Design review of the part shown in the three views and the two pictorial views. Dimensions are in mm from the part's minimum x, y and z. A direction names the side the tool comes from. Give positions to 0.01 mm unless a question says otherwise; leave off trailing zeros. Order: outer loops, then holes, each group sorted by start corner. A loop starts at its lowest first (then second) coordinate and runs counter-clockwise, first axis right, second up. Notation, with made-up numbers: (5.5, 54) - (43.5, 54) arc R35 cw to (43.5, 92) - close; hole circle Ø9 at (54, 58.25). An arc over 180 degrees is marked (long way). Put each result on its own line as item: value.
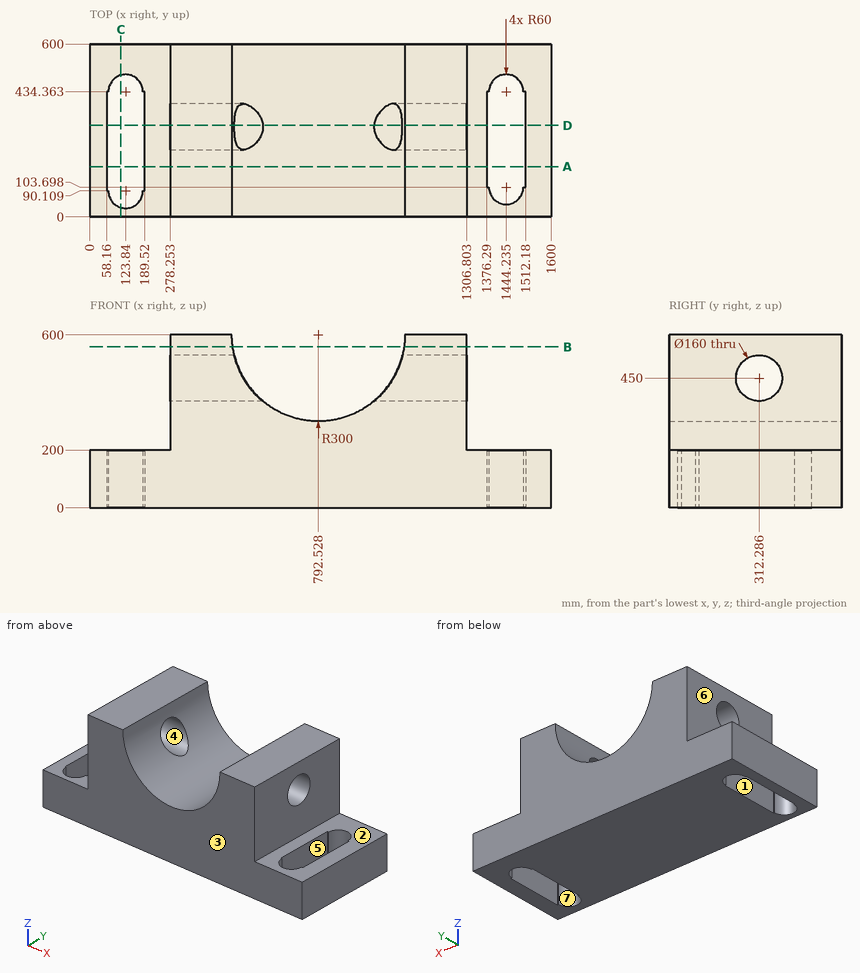
(1) For the marked faces 1, 2 and 3, list the 3-axis set-ups (+Z, -Z, +X, -X, +Y, -Y) from which the entire face can be reached by the end or side of a thin tool; tool diameter is ignored.
The answers:
face 1: +Z, -Z
face 2: +Z, +X, +Y, -Y
face 3: +Z, -Z, +X, -X, -Y
(2) Take a section at D-D, the plane y = 318. Write out the cut boundary in (x, z) (1 decimal), then the cut area to 3 significant figures.
The answers:
outline: (0, 0) - (58.2, 0) - (58.2, 200) - (0, 200) - close; (189.5, 0) - (1376.3, 0) - (1376.3, 200) - (1306.8, 200) - (1306.8, 370.2) - (985.4, 370.2) arc R300 cw to (599.7, 370.2) - (278.3, 370.2) - (278.3, 200) - (189.5, 200) - close; (278.3, 529.8) - (500.9, 529.8) arc R300 cw to (492.5, 600) - (278.3, 600) - close; (1084.2, 529.8) - (1306.8, 529.8) - (1306.8, 600) - (1092.5, 600) arc R300 cw to start; (1512.2, 0) - (1600, 0) - (1600, 200) - (1512.2, 200) - close
area: 454,000 mm^2
(3) Take a section at C-C, the plane x = 107. Write out the cut boundary in (y, z).
The answers:
outline: (0, 0) - (32.52, 0) - (32.52, 200) - (0, 200) - close; (491.95, 0) - (600, 0) - (600, 200) - (491.95, 200) - close
(4) Wall thickness on L1, parallel to X at y = 384, z = 186.5; L2, parallel to Y at x = 358, z = 450; L3, parallel to Y at x = 1440.5, z = 89.5 (1 decimal): over which ranges is each line inside the solid? List them lowest first.
The answers:
L1: 0 to 58.16, 189.52 to 1376.29, 1512.18 to 1600
L2: 0 to 232.29, 392.29 to 600
L3: 0 to 43.8, 494.2 to 600
(5) Take a section at B-B, the plane z = 558.5. Write out the cut boundary in (x, y), then the cut area to 3 significant figures.
The answers:
outline: (278.25, 0) - (495.41, 0) - (495.41, 600) - (278.25, 600) - close; (1089.64, 0) - (1306.8, 0) - (1306.8, 600) - (1089.64, 600) - close
area: 261,000 mm^2
(6) Clearance check with flat-ended pins moving along their axes: pin 1 Ø6 at (y, z) = (356, 281.5) entering from +X; pin 2 Ø3 at (y, z) = (169, 219.5) entering from -X; pin 3 Ø6 at (x, y) = (695.5, 157.5) entering from +Z. State where each tip first meets the part, or that it passes through.
The answers:
pin 1: x = 1306.8
pin 2: x = 278.25
pin 3: z = 317.17
(7) The part is to be moulded in two halves that separate along X. For the marked faces 4, 5, 6 and 7, say which applies: pulls with the +X half, pulls with the -X half, needs draft (parallel to the pull), parting line crosses it, or undercut.
The answers:
face 4: needs draft
face 5: undercut
face 6: pulls with the -X half
face 7: undercut
(8) Take a section at A-A, the plane y = 174.5. Write out the cut boundary in (x, z), then the cut area to 3 significant figures.
The answers:
outline: (0, 0) - (58.16, 0) - (58.16, 200) - (0, 200) - close; (189.52, 0) - (1376.29, 0) - (1376.29, 200) - (1306.8, 200) - (1306.8, 600) - (1092.53, 600) arc R300 cw to (492.53, 600) - (278.25, 600) - (278.25, 200) - (189.52, 200) - close; (1512.18, 0) - (1600, 0) - (1600, 200) - (1512.18, 200) - close
area: 537,000 mm^2
